Read the model definition and answer for the solid it produces. Units are mm, in the model's axes. A direction names the side the tool comes from. Round coordinates to 2 decimals unless told otherwise and drop trailing zeros. Order: outer loops, then holes, each group sorted by start corner. A loop starts at its lowest first (then second) coordinate and runs counter-clockwise, first axis right, second up. Notation, with made-up numbers: (-35.5, -1.75) -> (14.5, -1.75) arc R25 ccw to (14.5, 28.25) -> close; hole circle Ø6 at (54.25, 24.5). An arc over 180 degrees is marked (long way). Use a Markdown table: item, result. Add a question column.
1. For faces 1 (the face through (417.061, 334, 232)), 2 (the face through (418, 404.753, 127)), 3 (the face through (417.061, 204, 232)), determine the directions among +Z, -Z, +X, -X, +Y, -Y from which every point of the face is accessible in a straight line to the end or side of a thin tool.
2. Section C-C, the plane x = 184.5 is taken. Give the vertices of the cut face in (y, z), then the cut area to 3 significant figures.
3. Section B-B, the plane y = 360.5 is taken. Give the vertices of the cut face in (x, z).
4. Consider L1, parallel to Y at x = 383.5, z = 172; L2, parallel to Z at x = 5.5, y = 268; L3, parallel to X at y = 292.5, z = 85. Determine where each line is inside the solid, lowest interval first. Write a range as [from, to].
5. Section A-A, the plane z = 253.5 is taken. Give the vertices of the cut face in (x, y).
6. The mould has two halves that part along Y. Classify faces 4 (the face through (199, 4.753, 227)), 5 (the face through (199, 197, 0)), 6 (the face through (199, 202, 10)), 7 (the face through (204, 264.753, 232)): +Y half, -Y half, draft (parallel to the pull), parting line (faces both ways), or undercut.
7. Given pin 1 (10 mm diameter, centred on y = 315.5, z = 275, fed in from -X); pin 2 (5 mm diameter, centred on x = 303.5, y = -1.5, fed in from +Z); pin 3 (3 mm diameter, centred on x = 43, z = 385.5, fed in from +Y); pin 4 (10 mm diameter, centred on x = 205.5, y = 156, fed in from -Z), each flat-ended and moving along its own axis, determine where each tip first touches the part or whether it passes through.
8. Section D-D, the plane y = 65 is taken. Give the vertices of the cut face in (x, z), then the cut area to 3 significant figures.
```python
from build123d import *

# Parameters (mm, degrees)
SKETCH1_W           = 450
SKETCH1_H           = 10
BOSS_EXTRUDE1_DEPTH = 450
SKETCH2_W           = 450
SKETCH2_H           = 10
BOSS_EXTRUDE2_DEPTH = 400
SKETCH3_W           = 10
SKETCH3_H           = 250
BOSS_EXTRUDE3_DEPTH = 450
SKETCH4_W           = 420
SKETCH4_H           = 10
BOSS_EXTRUDE4_DEPTH = 450


with BuildPart() as part:
    # Sketch1 → Boss-Extrude1 (new body)
    with BuildSketch(Plane.XY):
        with Locations((202.060737527, -0.246746204)):
            Rectangle(SKETCH1_W, SKETCH1_H)
    extrude(amount=BOSS_EXTRUDE1_DEPTH)

    # Sketch2 → Boss-Extrude2 (add)
    with BuildSketch(Plane(origin=(0, 4.753253796, 0), x_dir=(1, 0, 0), z_dir=(0, 1, 0))):
        with Locations((202.060737527, -5)):
            Rectangle(SKETCH2_W, SKETCH2_H)
    extrude(amount=BOSS_EXTRUDE2_DEPTH)

    # Sketch3 → Boss-Extrude3 (add)
    with BuildSketch(Plane.XY.offset(10)):
        with Locations((422.060737527, 279.753253796)):
            Rectangle(SKETCH3_W, SKETCH3_H)
    extrude(amount=BOSS_EXTRUDE3_DEPTH)

    # Sketch4 → Boss-Extrude4 (add)
    with BuildSketch(Plane.XY.offset(10)):
        with Locations((207.060737527, 259.753253796)):
            Rectangle(SKETCH4_W, SKETCH4_H)
    extrude(amount=BOSS_EXTRUDE4_DEPTH)


solid = part.part
```
Verdict:
| question | item | result |
|---|---|---|
| 1 | face 1 | +Z, -X, +Y |
| 1 | face 2 | +Z, -Z, +X, -X, +Y |
| 1 | face 3 | +Z, -X |
| 2 | outline | (-5.25, 0) -> (404.75, 0) -> (404.75, 10) -> (264.75, 10) -> (264.75, 460) -> (254.75, 460) -> (254.75, 10) -> (4.75, 10) -> (4.75, 450) -> (-5.25, 450) -> close |
| 2 | area | 13,000 mm2 |
| 3 | outline | (-22.94, 0) -> (427.06, 0) -> (427.06, 460) -> (417.06, 460) -> (417.06, 10) -> (-22.94, 10) -> close |
| 4 | L1 | y = [-5.25, 4.75], [254.75, 264.75] |
| 4 | L2 | z = [0, 10] |
| 4 | L3 | x = [417.06, 427.06] |
| 5 | outline | (-22.94, -5.25) -> (427.06, -5.25) -> (427.06, 4.75) -> (-22.94, 4.75) -> close; (-2.94, 254.75) -> (417.06, 254.75) -> (417.06, 154.75) -> (427.06, 154.75) -> (427.06, 404.75) -> (417.06, 404.75) -> (417.06, 264.75) -> (-2.94, 264.75) -> close |
| 6 | face 4 | undercut |
| 6 | face 5 | draft |
| 6 | face 6 | undercut |
| 6 | face 7 | +Y half |
| 7 | pin 1 | stops at x = 417.06 |
| 7 | pin 2 | stops at z = 450 |
| 7 | pin 3 | stops at y = 264.75 |
| 7 | pin 4 | stops at z = 0 |
| 8 | outline | (-22.94, 0) -> (427.06, 0) -> (427.06, 10) -> (-22.94, 10) -> close |
| 8 | area | 4,500 mm2 |
